Source: CAD feature listing. Evaluate the final solid. Frame: model axes, mm. A direction names the side the tool comes from. Give positions to 0.01 mm unless a question says otherwise; leave off trailing zeros. Order: outer loops, then holes, each group sorted by start corner. A loop starts at its lowest first (then second) coordinate and runs counter-clockwise, first axis right, second up. Notation, with made-up numbers: (-33, 36.5) - (20, 36.5) arc R29 ccw to (20, 74.5) - close; hole circle Ø6 at (-7, 8.25). An arc over 180 degrees is marked (long way). One line per item, written item: value. Start each with the question number.
from build123d import *

# Parameters (mm, degrees)
SKETCH1_R               = 70
BOSS_EXTRUDE1_DEPTH     = 15
CUT_EXTRUDE5_DEPTH      = 55
CUT_EXTRUDE5_DEPTH_BACK = 101.124921973
SKETCH2_R               = 7
BOSS_EXTRUDE2_DEPTH     = 15
CIRPATTERN2_COUNT       = 20


with BuildPart() as part:
    # Sketch1 → Boss-Extrude1 (new body)
    with BuildSketch(Plane.XY):
        with Locations(Location((0, 0, 0), (0, 0, 180))):
            Circle(SKETCH1_R)
    extrude(amount=BOSS_EXTRUDE1_DEPTH)

    # Sketch2 → Cut-Extrude5 (cut, two sides: drawn at the far end of the back side and taken through both)
    with BuildSketch(Plane.XY.offset(-CUT_EXTRUDE5_DEPTH_BACK)):
        with Locations(Location((0, 0, 0), (0, 0, 180))):
            Circle(SKETCH2_R)
    extrude(amount=CUT_EXTRUDE5_DEPTH + CUT_EXTRUDE5_DEPTH_BACK, mode=Mode.SUBTRACT)

    # Sketch5 → Boss-Extrude2 (add)
    with BuildSketch(Plane.XY):
        Polygon((-6.539966856, 69.693822061), (-7.40050252, 78.864207898), (-2.856692059, 84.349096927), (2.856692059, 84.349096927), (7.40050252, 78.864207898), (6.539966856, 69.693822061), (6.538233044, 69.675345525), (-1.985773494, 69.971827928), (-6.526217216, 69.574369749), align=None)
    boss_extrude2 = extrude(amount=BOSS_EXTRUDE2_DEPTH)

    # CirPattern2: Boss-Extrude2 ×20 about axis
    cirpattern2_axis = Axis((0, 0, 0), (0, 0, 1))
    for i in range(1, CIRPATTERN2_COUNT):
        add(boss_extrude2.rotate(cirpattern2_axis, i * 360 / CIRPATTERN2_COUNT))


solid = part.part
1. Set-up query: faces 4 (the flat face through (81.645, -5.097, 7.395)), 5 (the cylindrical face through (31.835, 62.342, 7.395)), 6 (the flat face through (16.34, -72.86, 7.4)), 7 (the flat face through (-20.382, 79.224, 7.395)), 8 (the flat face through (-75.981, -30.114, 7.395)). Return all of +Z, -Z, +X, -X, +Y, -Y with unobstructed straight access to the full face (end or side cutting, diameter ignored); none if empty.
2. Draft query along Y for faces 1 (the flat face through (75.981, 30.114, 7.395)), 2 (the flat face through (-80.21, -26.1, 7.4)), 3 (the flat face through (79.224, 20.382, 7.395)). Return one class per face: pulls with the +Y half, pulls with the -Y half, needs draft (parallel to the pull), parting line crosses it, or undercut.
3. Section A-A on x = 0. Return the cut outline in (y, z), then the cut area to 3 significant figures.
4. Contact query for flat-ended pins moving along their axis: pin 1 Ø1.5 at (y, z) = (58, 5.5) entering from -X; pin 2 Ø3 at (x, z) = (24.5, 10) entering from -Y; pin 3 Ø1 at (y, z) = (27.5, 5.5) entering from +X. Output: stop coordinate, or through.
5. Ray query, L1, parallel to X at y = -50.5, z = 3.5; L2, parallel to X at y = -65.5, z = 1.5; L3, parallel to Y at x = -63, z = 10. Return the intervals inside material, ascending.
6. Section C-C on y = 20.5. Return the cut outline in (x, z), then the cut area to 3 significant figures.
Data:
1. face 4: +Z, -Z, +X
1. face 5: +Z, -Z
1. face 6: +Z, -Z, -Y
1. face 7: +Z, -Z, +Y
1. face 8: +Z, -Z, -X, -Y
2. face 1: pulls with the +Y half
2. face 2: pulls with the -Y half
2. face 3: undercut
3. outline: (-84.35, 0) - (-7, 0) - (-7, 15) - (-84.35, 15) - close; (7, 0) - (84.35, 0) - (84.35, 15) - (7, 15) - close
3. area: 2,320 mm2
4. pin 1: stops at x = -51.72
4. pin 2: stops at y = -81.1
4. pin 3: stops at x = 79.92
5. L1: x = -67.57 to -57.36, -48.47 to 48.47, 57.36 to 67.57
5. L2: x = -51.96 to -38.8, -28.29 to 28.29, 38.8 to 51.96
5. L3: y = -52.12 to -37.32, -30.51 to 30.51, 37.32 to 52.12
6. outline: (-79.3, 0) - (79.3, 0) - (79.3, 15) - (-79.3, 15) - close
6. area: 2,380 mm2
